```python
from build123d import *

# Parameters (mm, degrees)
SKETCH1_R           = 10
SKETCH1_R_2         = 6
BOSS_EXTRUDE1_DEPTH = 2
SKETCH2_R           = 9
BOSS_EXTRUDE2_DEPTH = 8
SKETCH3_R           = 5
BOSS_EXTRUDE3_DEPTH = 4
FILLET1_R           = 1


with BuildPart() as part:
    # Sketch1 → Boss-Extrude1 (new body)
    with BuildSketch(Plane(origin=(0, 0, 0), x_dir=(1, 0, 0), z_dir=(0, 1, 0))):
        with Locations(Location((0, 0, 0), (0, 0, 270))):
            Circle(SKETCH1_R)
        with Locations(Location((0, 0, 0), (0, 0, 270))):
            Circle(SKETCH1_R_2, mode=Mode.SUBTRACT)
    extrude(amount=BOSS_EXTRUDE1_DEPTH)

    # Sketch2 → Boss-Extrude2 (add)
    with BuildSketch(Plane(origin=(0, 0, 0), x_dir=(1, 0, 0), z_dir=(0, 1, 0))):
        with Locations(Location((0, 0, 0), (0, 0, 270))):
            Circle(SKETCH2_R)
    extrude(amount=-BOSS_EXTRUDE2_DEPTH)

    # Sketch3 → Boss-Extrude3 (add)
    with BuildSketch(Plane(origin=(0, 0, 0), x_dir=(1, 0, 0), z_dir=(0, 1, 0))):
        with Locations(Location((0, 0, 0), (0, 0, 270))):
            Circle(SKETCH3_R)
    extrude(amount=BOSS_EXTRUDE3_DEPTH)

    # Fillet1
    fillet1_edges = [part.edges().sort_by_distance(p)[0] for p in [
        (0, 4, -5),
        (0, 2, -10),
    ]]
    fillet(fillet1_edges, radius=FILLET1_R)


solid = part.part
```
Can you work these out from the model? Positions are in its coordinate system, mm. A direction names the side the tool comes from. Give positions to 0.01 mm unless a question says otherwise; leave off trailing zeros. Order: outer loops, then holes, each group sorted by start corner. A loop starts at its lowest first (then second) coordinate and runs counter-clockwise, first axis right, second up. Notation, with made-up numbers: M -15.75,65.25 L 19.25,65.25 A30 cw 19.25,88.25 Z; hole C -32,84.25 d3. An arc over 180 degrees is marked long. Write item = value, one per line. Start each with the question number.
Q1. Suppose I cut it at A-A (x = 0). Write out the boundary of the cut face in (y, z), plus the area to 3 significant figures.
Q2. I need wall thicknesses on probe 1 along X at (y, z) = (0.65, 0); probe 2 along X at (y, z) = (1.4, 0); probe 3 along Y at (x, z) = (-4.5, -7.75). Which ranges of each line are inside material? Lowest first, please. Write a range as [from, to].
Q3. For faces 1 (the cylindrical face through (-4.88, 1.48, -1.08)), 2 (the flat face through (2, 0, -9)), 3 (the flat face through (0, 4, 0)), which set-ups out of +Z, -Z, +X, -X, +Y, -Y let a thin tool reach every point of the face, with its end or its side?
Q4. Will these pins go through, and if not, where does the flat tip stop? pin 1 Ø1 at (y, z) = (-4, 3) entering from -X; pin 2 Ø4 at (y, z) = (0.5, -4.5) entering from -X; pin 3 Ø1.5 at (x, y) = (8, 0) entering from -Z.
Q5. Suppose I cut it at B-B (z = 0). Write out the boundary of the cut face in (x, y), plus the area to 3 significant figures.
Q6. We'd pull the mould along Z, two halves only. Please class faces 4 (the cylindrical face through (2.703, -3.944, 8.584)), 5 (the cylindrical face through (1.802, 0.986, 5.723)), 6 (the flat face through (0, -8, 0)): pulls with the +Z half, pulls with the -Z half, needs draft (parallel to the pull), parting line crosses it, or undercut.
Q7. Suppose I cut it at D-D (y = -6.25). Write out the boundary of the cut face in (x, z), plus the area to 3 significant figures.
Q8. Suppose I cut it at C-C (y = 1.5). Write out the boundary of the cut face in (x, z).
Check result:
q1.outline = M -8,-9 L 0,-9 L 0,-10 L 1,-10 A1 ccw 2,-9 L 2,-6 L 0,-6 L 0,-5 L 3,-5 A1 ccw 4,-4 L 4,4 A1 ccw 3,5 L 0,5 L 0,6 L 2,6 L 2,9 A1 ccw 1,10 L 0,10 L 0,9 L -8,9 Z
q1.area = 199 mm2
q2.probe_1 = [-10, -6], [-5, 5], [6, 10]
q2.probe_2 = [-9.92, -6], [-5, 5], [6, 9.92]
q2.probe_3 = [-8, 2]
q3.face_1 = +Y
q3.face_2 = -Y
q3.face_3 = +Z, -Z, +X, -X, +Y
q4.pin_1 = -8.65
q4.pin_2 = -9.68
q4.pin_3 = -6.89
q5.outline = M -10,0 L -9,0 L -9,-8 L 9,-8 L 9,0 L 10,0 L 10,1 A1 ccw 9,2 L 6,2 L 6,0 L 5,0 L 5,3 A1 ccw 4,4 L -4,4 A1 ccw -5,3 L -5,0 L -6,0 L -6,2 L -9,2 A1 ccw -10,1 Z
q5.area = 199 mm2
q6.face_4 = parting line crosses it
q6.face_5 = undercut
q6.face_6 = needs draft
q7.outline = C 0,0 d18
q7.area = 254 mm2
q8.outline = C 0,0 d19.73; C 0,0 d10; hole C 0,0 d12
